```python
from build123d import *

# Parameters (mm, degrees)
BOX035_W               = 60
BOX035_H               = 3
BOX035_DEPTH           = 11
BOX034_W               = 200
BOX034_H               = 30
BOX034_DEPTH           = 20
BOX033_W               = 60
BOX033_H               = 3
BOX033_DEPTH           = 11
BOX025_W               = 3
BOX025_H               = 20
BOX025_DEPTH           = 11
BOX026_W               = 3
BOX026_H               = 20
BOX026_DEPTH           = 11
BOX024_W               = 30
BOX024_H               = 20
BOX024_DEPTH           = 11
BOX023_W               = 20
BOX023_H               = 20
BOX023_DEPTH           = 11
CUT010_PLACEMENT_ANGLE = 180
BOX032_W               = 30
BOX032_H               = 20
BOX032_DEPTH           = 11
BOX031_W               = 20
BOX031_H               = 20
BOX031_DEPTH           = 11
CUT013_PLACEMENT_ANGLE = 180
BOX030_W               = 30
BOX030_H               = 20
BOX030_DEPTH           = 11
BOX029_W               = 20
BOX029_H               = 20
BOX029_DEPTH           = 11
CUT012_PLACEMENT_ANGLE = 180
BOX022_W               = 30
BOX022_H               = 20
BOX022_DEPTH           = 11
BOX021_W               = 20
BOX021_H               = 20
BOX021_DEPTH           = 11
CHAMFER006_SIZE        = 4
BOX018_W               = 178
BOX018_H               = 103.5
BOX018_DEPTH           = 30
BOX019_W               = 181
BOX019_H               = 121
BOX019_DEPTH           = 5
BOX017_W               = 186
BOX017_H               = 127
BOX017_DEPTH           = 4
FILLET008_R            = 2
FILLET009_R            = 1


with BuildPart() as cube032:
    # Box035 → Box035 (new body)
    with BuildSketch(Plane(origin=(63, 0, 4), x_dir=(1, 0, 0), z_dir=(0, 0, 1))):
        with Locations((30, 1.5)):
            Rectangle(BOX035_W, BOX035_H)
    extrude(amount=BOX035_DEPTH)


with BuildPart() as cube031:
    # Box034 → Box034 (new body)
    with BuildSketch(Plane(origin=(-10, 73, -5), x_dir=(1, 0, 0), z_dir=(0, 0, 1))):
        with Locations((100, 15)):
            Rectangle(BOX034_W, BOX034_H)
    extrude(amount=BOX034_DEPTH)


with BuildPart() as cube030:
    # Box033 → Box033 (new body)
    with BuildSketch(Plane(origin=(63, 112, 4), x_dir=(1, 0, 0), z_dir=(0, 0, 1))):
        with Locations((30, 1.5)):
            Rectangle(BOX033_W, BOX033_H)
    extrude(amount=BOX033_DEPTH)


with BuildPart() as cube022:
    # Box025 → Box025 (new body)
    with BuildSketch(Plane(origin=(0, 50, 4), x_dir=(1, 0, 0), z_dir=(0, 0, 1))):
        with Locations((1.5, 10)):
            Rectangle(BOX025_W, BOX025_H)
    extrude(amount=BOX025_DEPTH)


with BuildPart() as cube023:
    # Box026 → Box026 (new body)
    with BuildSketch(Plane(origin=(183, 50, 4), x_dir=(1, 0, 0), z_dir=(0, 0, 1))):
        with Locations((1.5, 10)):
            Rectangle(BOX026_W, BOX026_H)
    extrude(amount=BOX026_DEPTH)


with BuildPart() as cube021:
    # Box024 → Box024 (new body)
    with BuildSketch(Plane(origin=(3, 3, 0), x_dir=(1, 0, 0), z_dir=(0, 0, 1))):
        with Locations((15, 10)):
            Rectangle(BOX024_W, BOX024_H)
    extrude(amount=BOX024_DEPTH)


with BuildPart() as cut010:
    # Box023 → Box023 (new body)
    with BuildSketch(Plane.XY):
        with Locations((10, 10)):
            Rectangle(BOX023_W, BOX023_H)
    extrude(amount=BOX023_DEPTH)

    # Cut010: cut Cube021
    add(cube021.part, mode=Mode.SUBTRACT)


with BuildPart() as cut010_1:
    # Cut010 placement: moved
    add(cut010.part.moved(Location((186, 0, 15))).rotate(Axis((186, 0, 15), (0, 1, 0)), CUT010_PLACEMENT_ANGLE))


with BuildPart() as cube029:
    # Box032 → Box032 (new body)
    with BuildSketch(Plane(origin=(3, 3, 0), x_dir=(1, 0, 0), z_dir=(0, 0, 1))):
        with Locations((15, 10)):
            Rectangle(BOX032_W, BOX032_H)
    extrude(amount=BOX032_DEPTH)


with BuildPart() as cut013:
    # Box031 → Box031 (new body)
    with BuildSketch(Plane.XY):
        with Locations((10, 10)):
            Rectangle(BOX031_W, BOX031_H)
    extrude(amount=BOX031_DEPTH)

    # Cut013: cut Cube029
    add(cube029.part, mode=Mode.SUBTRACT)


with BuildPart() as cut013_1:
    # Cut013 placement: moved
    add(cut013.part.moved(Location((186, 115, 4))).rotate(Axis((186, 115, 4), (0, 0, 1)), CUT013_PLACEMENT_ANGLE))


with BuildPart() as cube027:
    # Box030 → Box030 (new body)
    with BuildSketch(Plane(origin=(3, 3, 0), x_dir=(1, 0, 0), z_dir=(0, 0, 1))):
        with Locations((15, 10)):
            Rectangle(BOX030_W, BOX030_H)
    extrude(amount=BOX030_DEPTH)


with BuildPart() as cut012:
    # Box029 → Box029 (new body)
    with BuildSketch(Plane.XY):
        with Locations((10, 10)):
            Rectangle(BOX029_W, BOX029_H)
    extrude(amount=BOX029_DEPTH)

    # Cut012: cut Cube027
    add(cube027.part, mode=Mode.SUBTRACT)


with BuildPart() as cut012_1:
    # Cut012 placement: moved
    add(cut012.part.moved(Location((0, 115, 15))).rotate(Axis((0, 115, 15), (1, 0, 0)), CUT012_PLACEMENT_ANGLE))


with BuildPart() as cube019:
    # Box022 → Box022 (new body)
    with BuildSketch(Plane(origin=(3, 3, 0), x_dir=(1, 0, 0), z_dir=(0, 0, 1))):
        with Locations((15, 10)):
            Rectangle(BOX022_W, BOX022_H)
    extrude(amount=BOX022_DEPTH)


with BuildPart() as chamfer006:
    # Box021 → Box021 (new body)
    with BuildSketch(Plane.XY):
        with Locations((10, 10)):
            Rectangle(BOX021_W, BOX021_H)
    extrude(amount=BOX021_DEPTH)

    # Cut009: cut Cube019
    add(cube019.part, mode=Mode.SUBTRACT)


with BuildPart() as chamfer006_1:
    # Cut009 placement: moved
    add(chamfer006.part.moved(Location((0, 0, 4))))

    # Fusion014: union Cube022, Cube023, Cut010, Cut013, Cut012
    add(cube022.part)
    add(cube023.part)
    add(cut010_1.part)
    add(cut013_1.part)
    add(cut012_1.part)

    # Fusion015: union Cube030
    add(cube030.part)

    # Cut014: cut Cube031
    add(cube031.part, mode=Mode.SUBTRACT)

    # Fusion016: union Cube032
    add(cube032.part)

    # Chamfer006
    chamfer006_edges = [chamfer006_1.edges().sort_by_distance(p)[0] for p in [
        (184.5, 20, 15),
        (166, 1.5, 15),
        (63, 113.5, 15),
        (123, 113.5, 15),
        (1.5, 103, 15),
        (20, 113.5, 15),
        (184.5, 50, 15),
        (184.5, 70, 15),
        (184.5, 103, 15),
        (166, 113.5, 15),
        (63, 1.5, 15),
        (123, 1.5, 15),
        (1.5, 50, 15),
        (1.5, 70, 15),
        (1.5, 20, 15),
        (20, 1.5, 15),
    ]]
    chamfer(chamfer006_edges, length=CHAMFER006_SIZE)


with BuildPart() as chamfer006_2:
    # Chamfer006 placement: moved
    add(chamfer006_1.part.moved(Location((0, 0, -1))))


with BuildPart() as cutout:
    # Box018 → Box018 (new body)
    with BuildSketch(Plane(origin=(4, 8, -25), x_dir=(1, 0, 0), z_dir=(0, 0, 1))):
        with Locations((89, 51.75)):
            Rectangle(BOX018_W, BOX018_H)
    extrude(amount=BOX018_DEPTH)


with BuildPart() as cube016:
    # Box019 → Box019 (new body)
    with BuildSketch(Plane(origin=(2.5, 3, -5), x_dir=(1, 0, 0), z_dir=(0, 0, 1))):
        with Locations((90.5, 60.5)):
            Rectangle(BOX019_W, BOX019_H)
    extrude(amount=BOX019_DEPTH)


with BuildPart() as fascia_modified:
    # Box017 → Box017 (new body)
    with BuildSketch(Plane.XY):
        with Locations((93, 63.5)):
            Rectangle(BOX017_W, BOX017_H)
    extrude(amount=BOX017_DEPTH)

    # Fusion007: union Cube016
    add(cube016.part)

    # Cut007: cut Cutout
    add(cutout.part, mode=Mode.SUBTRACT)

    # Fillet008
    fillet008_edges = [fascia_modified.edges().sort_by_distance(p)[0] for p in [
        (183.5, 124, -2.5),
        (2.5, 124, -2.5),
        (2.5, 3, -2.5),
        (183.5, 3, -2.5),
    ]]
    fillet(fillet008_edges, radius=FILLET008_R)

    # Fillet009
    fillet009_edges = [fascia_modified.edges().sort_by_distance(p)[0] for p in [
        (93, 124, -5),
        (3.085786, 123.414214, -5),
        (182.914214, 123.414214, -5),
        (2.5, 63.5, -5),
        (183.5, 63.5, -5),
        (3.085786, 3.585786, -5),
        (182.914214, 3.585786, -5),
        (93, 3, -5),
    ]]
    fillet(fillet009_edges, radius=FILLET009_R)

    # Fusion017: union Chamfer006
    add(chamfer006_2.part)


solid = fascia_modified.part
```
The listing builds one solid part. Answer for the finished solid, in the listing's coordinates (mm). A direction names the side the tool comes from. Coordinates: 2 decimals unless noted, no trailing zeros. Write each loop counter-clockwise with the first axis right and the second up, starting at its lowest first coordinate (ties: lowest second). Pieces come first, ordered by that corner, then holes.
Q1. Find the intervals of material crossed by line 1 along Y through (x, z) = (117, 11.5); line 2 along X through (y, z) = (99.5, -2); line 3 along Y through (x, z) = (104.5, 1.75), in increasing order.
Returned:
line 1: y = 0 to 3, 112 to 115
line 2: x = 2.5 to 4, 182 to 183.5
line 3: y = 0 to 8, 111.5 to 127
Q2. Which of the six approach directions +Z, -Z, +X, -X, +Y, -Y give full straight-line access (tool end or side, diameter ignored) to faces 4 (the flat face through (92, 111.5, -1)), 5 (the flat face through (175, 3, 9)), 6 (the flat face through (18, 114, 12))?
Returned:
face 4: +Z, -Z
face 5: +Z
face 6: +Z, +Y, -Y
Q3. Section A-A, the plane x = 99 is taken. Write down the section's boundary in (y, z).
Returned:
outline: (0, 0) - (3, 0) - (3, -4) arc R1 ccw to (4, -5) - (8, -5) - (8, 4) - (3, 4) - (3, 14) - (0, 14) - close; (111.5, -5) - (123, -5) arc R1 ccw to (124, -4) - (124, 0) - (127, 0) - (127, 4) - (115, 4) - (115, 14) - (112, 14) - (112, 4) - (111.5, 4) - close
Q4. Section B-B, the plane y = 56 is taken. Write down the section's boundary in (x, z), then the cut area to 3 significant figures.
Returned:
outline: (0, 0) - (2.5, 0) - (2.5, -4) arc R1 ccw to (3.5, -5) - (4, -5) - (4, 4) - (3, 4) - (3, 14) - (0, 14) - close; (182, -5) - (182.5, -5) arc R1 ccw to (183.5, -4) - (183.5, 0) - (186, 0) - (186, 14) - (183, 14) - (183, 4) - (182, 4) - close
area: 107 mm2
Q5. Section C-C, the plane x = 31 is taken. Write down the section's boundary in (y, z), then the cut area to 3 significant figures.
Returned:
outline: (0, 0) - (3, 0) - (3, -4) arc R1 ccw to (4, -5) - (8, -5) - (8, 4) - (0, 4) - close; (111.5, -5) - (123, -5) arc R1 ccw to (124, -4) - (124, 0) - (127, 0) - (127, 4) - (111.5, 4) - close
area: 181 mm2
Q6. The mould has two halves that part along Y. Classify faces 1 (the flat face through (3, 108, 9)), 2 (the flat face through (92, 0, 5)), 3 (the flat face through (186, 63, 5)): released by +Y, released by -Y, zero draft, split by the parting line, or undercut.
Returned:
face 1: undercut
face 2: released by -Y
face 3: zero draft
Q7. Given P1, Ø8, axis at x = 175.5, z = 8.5, coming from the +Y side, flat-ended and moving along its own axis, determine where the tip first touches the part or whether it passes through.
Returned:
P1: stops at y = 115
Q8. Section D-D, the plane z = 6.5 is taken. Give the number of separate pieces and of enclosed holes in the cut face, then the cut area to 3 significant figures.
Returned:
separate pieces: 8
enclosed holes: 0
area: 876 mm2
